Geometry check sheet. Reference: the model listing, model coordinates, mm. A direction names the side the tool comes from. Round coordinates to 2 decimals unless told otherwise and drop trailing zeros. Write each loop counter-clockwise with the first axis right and the second up, starting at its lowest first coordinate (ties: lowest second). Pieces come first, ordered by that corner, then holes. Notation, with made-up numbers: (-30, 34) - (14, 34) arc R14 cw to (14, 59) - close; hole circle Ø9 at (34.5, -24). An arc over 180 degrees is marked (long way). Return JSON: item names as keys, results as strings.
```python
from build123d import *

# Parameters (mm, degrees)
PAD017_DEPTH    = 3.5
POCKET027_DEPTH = 2
SKETCH054_W     = 34
SKETCH054_H     = 4.8
PAD020_DEPTH    = 1.5
PAD021_DEPTH    = 1.5
SKETCH049_W     = 4
SKETCH049_H     = 17.5
POCKET028_DEPTH = 0.5
POCKET029_DEPTH = 0.8


with BuildPart() as part:
    # Sketch045 → Pad017 (new body)
    with BuildSketch(Plane.XY):
        with BuildLine():
            ThreePointArc((-23, 23.3), (-23.9192388155, 22.9192388155), (-24.3, 22))
            Line((-24.3, 22), (-24.3, 17.1))
            Line((-26, 17.1), (-24.3, 17.1))
            Line((-26, -16.9), (-26, 17.1))
            Line((-24.3, -16.9), (-26, -16.9))
            Line((-24.3, -16.9), (-24.3, -22))
            ThreePointArc((-24.3, -22), (-23.9192388155, -22.9192388155), (-23, -23.3))
            Line((-21.3, -23.3), (-23, -23.3))
            Line((-21.3, -25.3), (-21.3, -23.3))
            Line((-22, -25.3), (-21.3, -25.3))
            Line((-22, -27.2), (-22, -25.3))
            ThreePointArc((-22, -27.2), (-20.5355339059, -30.7355339059), (-17, -32.2))
            Line((-17, -32.2), (17, -32.2))
            ThreePointArc((17, -32.2), (20.5355339059, -30.7355339059), (22, -27.2))
            Line((22, -27.2), (22, -25.3))
            Line((22, -25.3), (21.3, -25.3))
            Line((21.3, -25.3), (21.3, -23.3))
            Line((21.3, -23.3), (23, -23.3))
            ThreePointArc((23, -23.3), (23.9192388155, -22.9192388155), (24.3, -22))
            Line((24.3, -22), (24.3, -10.7))
            Line((26, -10.7), (24.3, -10.7))
            Line((26, 17.2), (26, -10.7))
            Line((24.3, 17.2), (26, 17.2))
            Line((24.3, 22), (24.3, 17.2))
            ThreePointArc((24.3, 22), (23.9192388155, 22.9192388155), (23, 23.3))
            Line((21.3, 23.3), (23, 23.3))
            Line((21.3, 25.3), (21.3, 23.3))
            Line((22, 25.3), (21.3, 25.3))
            Line((22, 27.2), (22, 25.3))
            ThreePointArc((22, 27.2), (20.5355339059, 30.7355339059), (17, 32.2))
            Line((-17, 32.2), (17, 32.2))
            ThreePointArc((-17, 32.2), (-20.5355339059, 30.7355339059), (-22, 27.2))
            Line((-22, 27.2), (-22, 25.3))
            Line((-22, 25.3), (-21.3, 25.3))
            Line((-21.3, 25.3), (-21.3, 23.3))
            Line((-21.3, 23.3), (-23, 23.3))
        make_face()
        with BuildLine():
            ThreePointArc((-17, 28.7), (-18.5, 27.2), (-17, 25.7))
            Line((-17, 25.7), (-5, 25.7))
            ThreePointArc((-5, 25.7), (-3.5, 27.2), (-5, 28.7))
            Line((-17, 28.7), (-5, 28.7))
        make_face(mode=Mode.SUBTRACT)
        with BuildLine():
            ThreePointArc((5, 28.7), (3.5, 27.2), (5, 25.7))
            Line((5, 25.7), (17, 25.7))
            ThreePointArc((17, 25.7), (18.5, 27.2), (17, 28.7))
            Line((5, 28.7), (17, 28.7))
        make_face(mode=Mode.SUBTRACT)
        with BuildLine():
            ThreePointArc((-17, -25.7), (-18.5, -27.2), (-17, -28.7))
            Line((-17, -28.7), (-5, -28.7))
            ThreePointArc((-5, -28.7), (-3.5, -27.2), (-5, -25.7))
            Line((-17, -25.7), (-5, -25.7))
        make_face(mode=Mode.SUBTRACT)
        with BuildLine():
            ThreePointArc((5, -25.7), (3.5, -27.2), (5, -28.7))
            Line((5, -28.7), (17, -28.7))
            ThreePointArc((17, -28.7), (18.5, -27.2), (17, -25.7))
            Line((5, -25.7), (17, -25.7))
        make_face(mode=Mode.SUBTRACT)
    extrude(amount=PAD017_DEPTH)

    # Sketch047 (on Face53 of Pad017) → Pocket027 (cut)
    with BuildSketch(Plane(origin=(0, 0, 0), x_dir=(1, 0, 0), z_dir=(0, 0, -1))):
        Polygon((20.5, -23.3), (-20.5, -23.3), (-20.5, -20.3), (-26, -20.3), (-26, 20.3), (-20.5, 20.3), (-20.5, 23.3), (20.5, 23.3), (20.5, 20.3), (26, 20.3), (26, -20.3), (20.5, -20.3), align=None)
    extrude(amount=-POCKET027_DEPTH, mode=Mode.SUBTRACT)

    # Sketch054 (on Face32 of Pocket027) → Pad020 (join)
    with BuildSketch(Plane(origin=(-26, 0, 0), x_dir=(0, -1, 0), z_dir=(-1, 0, 0))):
        with Locations((-0.1, 1.1)):
            Rectangle(SKETCH054_W, SKETCH054_H)
    extrude(amount=-PAD020_DEPTH)

    # Sketch055 (on Face31 of Pad020) → Pad021 (join)
    with BuildSketch(Plane.YZ.offset(26)):
        Polygon((1.8, 3.5), (1.8, 0), (8.8, 0), (8.8, -1.5), (17.2, -1.5), (17.2, 3.5), align=None)
    extrude(amount=-PAD021_DEPTH)

    # Sketch049 (on Face49 of Pad021) → Pocket028 (cut)
    with BuildSketch(Plane(origin=(0, 0, 2), x_dir=(1, 0, 0), z_dir=(0, 0, -1))):
        with Locations((-22.5, 0.25)):
            Rectangle(SKETCH049_W, SKETCH049_H)
    extrude(amount=-POCKET028_DEPTH, mode=Mode.SUBTRACT)

    # Sketch048 (on Face4 of Pocket028) → Pocket029 (cut)
    with BuildSketch(Plane.XY.offset(3.5)):
        with BuildLine():
            ThreePointArc((24.3, 22), (23.9192388155, 22.9192388155), (23, 23.3))
            Line((23, 23.3), (21.3, 23.3))
            Line((21.3, 23.3), (21.3, 22.7))
            Line((21.3, 22.7), (23.0000081541, 22.7))
            ThreePointArc((23.7, 22.0000000128), (23.4949776252, 22.4949718684), (23.0000081541, 22.7))
            Line((23.7, 22.0000000128), (23.7, 17.2))
            Line((23.7, 17.2), (24.3, 17.2))
            Line((24.3, 17.2), (24.3, 22))
        make_face()
        with BuildLine():
            Line((23, -23.3), (21.3, -23.3))
            Line((21.3, -23.3), (21.3, -22.7))
            Line((21.3, -22.7), (23.0000012126, -22.7))
            ThreePointArc((23.0000012126, -22.7), (23.4949754721, -22.4949748266), (23.7, -22.0000002998))
            Line((23.7, -10.7), (23.7, -22.0000002998))
            Line((23.7, -10.7), (24.3, -10.7))
            Line((24.3, -10.7), (24.3, -22))
            ThreePointArc((23, -23.3), (23.9192392181, -22.9192392181), (24.3, -22))
        make_face()
        with BuildLine():
            ThreePointArc((-23, 23.3), (-23.9192388155, 22.9192388155), (-24.3, 22))
            Line((-24.3, 22), (-24.3, 17.1))
            Line((-24.3, 17.1), (-23.7, 17.1))
            Line((-23.7, 17.1), (-23.7, 21.9999998829))
            ThreePointArc((-23, 22.7), (-23.4949747882, 22.4949747054), (-23.7, 21.9999998829))
            Line((-23, 22.7), (-21.3, 22.7))
            Line((-21.3, 22.7), (-21.3, 23.3))
            Line((-21.3, 23.3), (-23, 23.3))
        make_face()
        with BuildLine():
            ThreePointArc((-24.3, -22), (-23.9192388155, -22.9192388155), (-23, -23.3))
            Line((-23, -23.3), (-21.3, -23.3))
            Line((-21.3, -23.3), (-21.3, -22.7))
            Line((-21.3, -22.7), (-23.0000001118, -22.7))
            ThreePointArc((-23.7, -22), (-23.4949747864, -22.4949747073), (-23.0000001118, -22.7))
            Line((-23.7, -22), (-23.7, -16.9))
            Line((-23.7, -16.9), (-24.3, -16.9))
            Line((-24.3, -16.9), (-24.3, -22))
        make_face()
    extrude(amount=-POCKET029_DEPTH, mode=Mode.SUBTRACT)


with BuildPart() as part_1:
    # Body004 placement: moved
    add(part.part.moved(Location((0, 0, -0.5))))


solid = part_1.part
```
(1) Material ranges on line 1 along Y through (x, z) = (-12, 1.45); line 2 along Y through (x, z) = (17.5, 2.1); line 3 along Z through (x, y) = (-17.5, -3.5), recorded low to high. Write a range as [from, to].
Response values:
{"line 1": "y = [-32.2, -28.7], [-25.7, -23.3], [23.3, 25.7], [28.7, 32.2]", "line 2": "y = [-32.17, -28.61], [-25.79, 25.79], [28.61, 32.17]", "line 3": "z = [1.5, 3]"}
(2) Section check A-A, the plane x = -10.5. Enter the section's corners in (y, z), plus the area to 3 significant figures.
Response values:
{"outline": "(-32.2, -0.5) - (-28.7, -0.5) - (-28.7, 3) - (-32.2, 3) - close; (-25.7, -0.5) - (-23.3, -0.5) - (-23.3, 1.5) - (23.3, 1.5) - (23.3, -0.5) - (25.7, -0.5) - (25.7, 3) - (-25.7, 3) - close; (28.7, -0.5) - (32.2, -0.5) - (32.2, 3) - (28.7, 3) - close", "area": "111 mm^2"}
(3) Section check C-C, the plane y = -3.5. Enter the section's corners in (x, z), plus the area to 4 significant figures.
Response values:
{"outline": "(-26, -1.8) - (-24.5, -1.8) - (-24.5, 2) - (-20.5, 2) - (-20.5, 1.5) - (26, 1.5) - (26, 3) - (-26, 3) - close", "area": "80.95 mm^2"}
(4) Release check for a two-part mould opening along X. For faces 1 (the face through (23.93, 22.91, 0.83)), 2 (the face through (-20.5, 30.77, 1.23)), 3 (the face through (-20.5, -22, 0)) record: pulls with the +X half, pulls with the -X half, needs draft (parallel to the pull), parting line crosses it, or undercut.
Response values:
{"face 1": "pulls with the +X half", "face 2": "pulls with the -X half", "face 3": "undercut"}
(5) Access from +Z, -Z, +X, -X, +Y, -Y to the whole of each face (thin tool, end or side, straight path). Record for faces 4 (the face through (-20.5, 22, 0)), 5 (the face through (-24.3, 21, 1)), 6 (the face through (-22, -26, 1)), 7 (the face through (26, 7, 1)), 8 (the face through (-26, 0, 1)).
Response values:
{"face 4": "-Z", "face 5": "+Z, -Z, -X, +Y", "face 6": "+Z, -Z, -X, -Y", "face 7": "+Z, -Z, +X, +Y, -Y", "face 8": "+Z, -Z, -X, +Y, -Y"}
(6) Section check B-B, the plane z = 0.4. Give the number of separate pieces and of enclosed holes in the cut face, plus the area to 3 significant figures.
Response values:
{"separate pieces": "4", "enclosed holes": "4", "area": "702 mm^2"}
(7) Gauge pin test, flat ends, axial feed: pin 1 (9.5 mm diameter, centred on x = -5.5, y = -24, fed in from -Z); pin 2 (1.5 mm diameter, centred on y = 26.5, z = 1.5, fed in from -X); pin 3 (3 mm diameter, centred on y = 24.5, z = 1, fed in from -X). Record the tip position at first contact, or that the pin passes through.
Response values:
{"pin 1": "stops at z = -0.5", "pin 2": "stops at x = -22", "pin 3": "stops at x = -23.83"}
